Work out the finished part from the listing and answer in its coordinate system (mm). Face numbers are marked on the shaded views. A direction names the side the tool comes from. Round coordinates to 2 decimals unless told otherwise and drop trailing zeros. Write each loop counter-clockwise with the first axis right and the second up, starting at its lowest first coordinate (ties: lowest second). Pieces come first, ordered by that corner, then holes. Notation, with made-up numbers: (-21, 58.25) - (-14, 58.25) arc R22 cw to (-14, 89.25) - close; hole circle Ø1 at (-7, 34). An arc over 180 degrees is marked (long way). Answer as a JSON object with one key per item and string values.
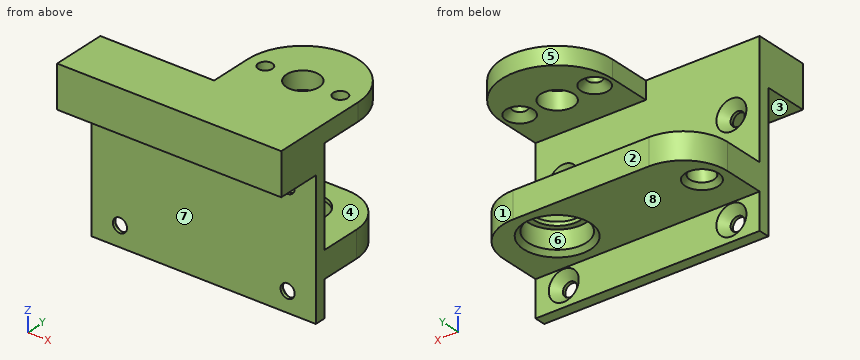
```python
from build123d import *

# Parameters (mm, degrees)
PAD016_DEPTH    = 4
SKETCH074_W     = 50.8
SKETCH074_H     = 2.5
PAD017_DEPTH    = 36.1
SKETCH082_W     = 50.8
SKETCH082_H     = 10
PAD018_DEPTH    = 5.5
SKETCH075_R     = 3.7
POCKET065_DEPTH = 5
SKETCH076_R     = 1.6
POCKET066_DEPTH = 5
SKETCH077_W     = 50.8
SKETCH077_H     = 6
PAD019_DEPTH    = 19.27
SKETCH078_R     = 6.585
POCKET067_DEPTH = 5.1625
SKETCH079_R     = 5.25
POCKET068_DEPTH = 5
SKETCH080_R     = 2.75
POCKET069_DEPTH = 4
SKETCH081_R     = 1.6
POCKET070_DEPTH = 5
CHAMFER010_SIZE = 1.8
CHAMFER011_SIZE = 1
CHAMFER012_SIZE = 1.5
FILLET001_R     = 10


with BuildPart() as part:
    # Sketch073 → Pad016 (new body)
    with BuildSketch(Plane.XY):
        with BuildLine():
            Line((-25.4, 2.5), (-25.4, -10))
            Line((-25.4, -10), (25.4, -10))
            Line((25.4, -10), (25.4, 2.5))
            Line((25.4, 2.5), (25.4, 12.185))
            ThreePointArc((25.4, 12.185), (12.9, 24.685), (0.4, 12.185))
            Line((0.4, 2.5), (0.4, 12.185))
            Line((0.4, 2.5), (-25.4, 2.5))
        make_face()
    extrude(amount=PAD016_DEPTH)

    # Sketch074 (on Face8 of Pad016) → Pad017 (join)
    with BuildSketch(Plane(origin=(0, 0, 0), x_dir=(1, 0, 0), z_dir=(0, 0, -1))):
        with Locations((0, -1.25)):
            Rectangle(SKETCH074_W, SKETCH074_H)
    extrude(amount=PAD017_DEPTH)

    # Sketch082 (on Face5 of Pad017) → Pad018 (join)
    with BuildSketch(Plane(origin=(0, 0, 0), x_dir=(1, 0, 0), z_dir=(0, 0, -1))):
        with Locations((0, 5)):
            Rectangle(SKETCH082_W, SKETCH082_H)
    extrude(amount=PAD018_DEPTH)

    # Sketch075 → Pocket065 (cut)
    with BuildSketch(Plane.XY.offset(4)):
        with Locations((12.9, 12.185)):
            Circle(SKETCH075_R)
    extrude(amount=-POCKET065_DEPTH, mode=Mode.SUBTRACT)

    # Sketch076 → Pocket066 (cut)
    with BuildSketch(Plane(origin=(0, 2.5, 0), x_dir=(-1, 0, 0), z_dir=(0, 1, 0))):
        with Locations((-19, -10)):
            Circle(SKETCH076_R)
        with Locations((19, -10)):
            Circle(SKETCH076_R)
        with Locations((19, -31.575)):
            Circle(SKETCH076_R)
        with Locations((-19, -31.575)):
            Circle(SKETCH076_R)
    extrude(amount=-POCKET066_DEPTH, mode=Mode.SUBTRACT)

    # Sketch077 → Pad019 (join)
    with BuildSketch(Plane(origin=(0, 2.5, 0), x_dir=(-1, 0, 0), z_dir=(0, 1, 0))):
        with Locations((0, -25)):
            Rectangle(SKETCH077_W, SKETCH077_H)
    extrude(amount=PAD019_DEPTH)

    # Sketch078 (on Face27 of Pad019) → Pocket067 (cut)
    with BuildSketch(Plane(origin=(0, 0, -28), x_dir=(1, 0, 0), z_dir=(0, 0, -1))):
        with Locations((12.9, -12.185)):
            Circle(SKETCH078_R)
    extrude(amount=-POCKET067_DEPTH, mode=Mode.SUBTRACT)

    # Sketch079 (on Face31 of Pocket067) → Pocket068 (cut)
    with BuildSketch(Plane(origin=(0, 0, -22.8375), x_dir=(1, 0, 0), z_dir=(0, 0, -1))):
        with Locations((12.9, -12.185)):
            Circle(SKETCH079_R)
    extrude(amount=-POCKET068_DEPTH, mode=Mode.SUBTRACT)

    # Sketch080 (on Face27 of Pocket068) → Pocket069 (cut)
    with BuildSketch(Plane(origin=(0, 0, -28), x_dir=(1, 0, 0), z_dir=(0, 0, -1))):
        with Locations((-19.9, -12.185)):
            Circle(SKETCH080_R)
    extrude(amount=-POCKET069_DEPTH, mode=Mode.SUBTRACT)

    # Sketch081 → Pocket070 (cut)
    with BuildSketch(Plane.XY.offset(4)):
        with Locations((4.4, 12.185)):
            Circle(SKETCH081_R)
        with Locations((21.4, 12.185)):
            Circle(SKETCH081_R)
    extrude(amount=-POCKET070_DEPTH, mode=Mode.SUBTRACT)

    # Chamfer010
    chamfer010_edges = [part.edges().sort_by_distance(p)[0] for p in [
        (20.6, 2.5, -31.575),
        (-17.4, 2.5, -31.575),
        (20.6, 2.5, -10),
        (-17.4, 2.5, -10),
    ]]
    chamfer(chamfer010_edges, length=CHAMFER010_SIZE)

    # Chamfer011
    chamfer011_edges = [part.edges().sort_by_distance(p)[0] for p in [
        (6.315, 12.185, -28),
        (-22.65, 12.185, -28),
    ]]
    chamfer(chamfer011_edges, length=CHAMFER011_SIZE)

    # Chamfer012
    chamfer012_edges = [part.edges().sort_by_distance(p)[0] for p in [
        (19.8, 12.185, 0),
        (2.8, 12.185, 0),
    ]]
    chamfer(chamfer012_edges, length=CHAMFER012_SIZE)

    # Fillet001
    fillet001_edges = [part.edges().sort_by_distance(p)[0] for p in [
        (25.4, 21.77, -25),
        (-25.4, 21.77, -25),
    ]]
    fillet(fillet001_edges, radius=FILLET001_R)


solid = part.part
```
Item 1: Determine the mould class of the marked faces 6, 7 and 8 for opening direction Y: pulls with the +Y half, pulls with the -Y half, needs draft (parallel to the pull), parting line crosses it, or undercut.
Results found:
{"face 6": "undercut", "face 7": "pulls with the -Y half", "face 8": "needs draft"}
Item 2: A cutting plane is placed at C-C (x = 12.9). Write down the section's boundary in (y, z) (1 decimal), and give its area (3 significant figures).
Results found:
{"outline": "(-10, -5.5) - (0, -5.5) - (0, -36.1) - (2.5, -36.1) - (2.5, -28) - (4.6, -28) - (5.6, -27) - (5.6, -22.8) - (6.9, -22.8) - (6.9, -22) - (2.5, -22) - (2.5, 0) - (8.5, 0) - (8.5, 4) - (-10, 4) - close; (15.9, 0) - (24.7, 0) - (24.7, 4) - (15.9, 4) - close; (17.4, -22.8) - (18.8, -22.8) - (18.8, -27) - (19.8, -28) - (21.8, -28) - (21.8, -22) - (17.4, -22) - close", "area": "292 mm²"}
Item 3: A cutting plane is placed at D-D (z = -3.5). Write down the section's boundary in (x, y), and give its area (3 significant figures).
Results found:
{"outline": "(-25.4, -10) - (25.4, -10) - (25.4, 2.5) - (-25.4, 2.5) - close", "area": "635 mm²"}
Item 4: For the marked faces 1, 2, 3, 4 and 5, determine the directions among +Z, -Z, +X, -X, +Y, -Y from which every point of the face is accessible in a straight line to the end or side of a thin tool.
Results found:
{"face 1": "-Z, +X, +Y", "face 2": "-Z, +X, -X, +Y", "face 3": "-Z, +X, -X, -Y", "face 4": "+X, -X, +Y", "face 5": "+Z, +Y"}
Item 5: Consider line 1 along Z through (x, y) = (20, 5); line 2 along Z through (x, y) = (-21, 4.5); line 3 along Y through (x, z) = (-9.5, -32.5). Determine where each line is inside the solid, lowest interval first.
Results found:
{"line 1": "-28 to -22, 0 to 4", "line 2": "-28 to -22", "line 3": "0 to 2.5"}
Item 6: A cutting plane is placed at B-B (x = -10). Write down the section's boundary in (y, z).
Results found:
{"outline": "(-10, -5.5) - (0, -5.5) - (0, -36.1) - (2.5, -36.1) - (2.5, -28) - (21.77, -28) - (21.77, -22) - (2.5, -22) - (2.5, 4) - (-10, 4) - close"}
Item 7: Each of these flat-tipped pins is pushed along its axis until it touches: P1, Ø4, axis at x = -1.5, y = 21, coming from the +Z side; P2, Ø12, axis at x = 12.9, y = 12.185, coming from the -Z side; P3, Ø3.5, axis at x = -19, z = -31.575, coming from the -Y side; P4, Ø4.5, axis at x = 12.9, y = 12.185, coming from the -Z side. Where does it stop, or does it pass through?
Results found:
{"P1": "z = -22", "P2": "z = -22.84", "P3": "y = 0", "P4": "through"}
Item 8: A cutting plane is placed at A-A (z = -10). Write down the section's boundary in (x, y).
Results found:
{"outline": "(-25.4, 0) - (-20.6, 0) - (-20.6, 0.7) - (-22.4, 2.5) - (-25.4, 2.5) - close; (-17.4, 0) - (17.4, 0) - (17.4, 0.7) - (15.6, 2.5) - (-15.6, 2.5) - (-17.4, 0.7) - close; (20.6, 0) - (25.4, 0) - (25.4, 2.5) - (22.4, 2.5) - (20.6, 0.7) - close"}
